The model under review builds one solid part; all positions refer to its coordinate system, in mm. A direction names the side the tool comes from. Coordinates: 2 decimals unless noted, no trailing zeros. Loops run counter-clockwise (first coordinate to the right, second up) from the corner with the lowest first, then second, coordinate; pieces in that order, holes last. Notation, with made-up numbers: M 88.25,-19.5 L 99.25,-19.5 A15 cw 99.25,8.5 Z; hole C 76.5,-8 d10. An arc over 180 degrees is marked long. Write item = value, one per line. Start each with the question number.
Q1. Clearance check with flat-ended pins moving along their axes: pin 1 Ø5 at (x, y) = (39, 3) entering from +Z; pin 2 Ø10 at (x, z) = (27, 9) entering from +Y; pin 3 Ø9.5 at (x, z) = (71, 0.5) entering from -Y. State where each tip first meets the part, or that it passes through.
Q2. For faces 4 (the face through (77, 19, 6.5)), 5 (the face through (-8, -5, 9)), 6 (the face through (-15.62, 14.6, -3.47)), 7 (the face through (36, 5, -6.5)), list the 3-axis set-ups (+Z, -Z, +X, -X, +Y, -Y) from which the entire face can be reached by the end or side of a thin tool; tool diameter is ignored.
Q3. Mouldability with a two-part tool opening along X and no side actions: class faces 1 (the face through (28.885, 8.019, 5.899)), 2 (the face through (78.64, 23.09, -0.09)), 3 (the face through (0, 0, -13)) as released by +X, released by -X, zero draft, split by the parting line, or undercut.
Q4. We need section A-A on y = -20.5. Give the boundary of the cut face in (x, z).
Q5. We need section C-C on y = 32.5. Give the boundary of the cut face in (x, z), and give its area (3 significant figures).
Q6. Wall thickness on probe 1 along X at (y, z) = (19, 0); probe 2 along X at (y, z) = (16, 0); probe 3 along Y at (x, z) = (0, 3): over which ranges is each line inside the solid? List them lowest first.
Q7. We need section B-B on y = 83. Give the boundary of the cut face in (x, z).
from build123d import *

# Parameters (mm, degrees)
SKETCH1_R           = 21
BOSS_EXTRUDE1_DEPTH = 22
SKETCH3_W           = 35
SKETCH3_H           = 18
BOSS_EXTRUDE2_DEPTH = 15
BOSS_EXTRUDE3_DEPTH = 9
SKETCH6_R           = 12.5
CUT_EXTRUDE1_DEPTH  = 18
BOSS_EXTRUDE5_DEPTH = 6.5
SKETCH9_R           = 20
BOSS_EXTRUDE6_DEPTH = 55
SKETCH10_R          = 22.5
BOSS_EXTRUDE7_DEPTH = 33
FILLET1_R           = 15
CHAMFER2_SIZE       = 10
FILLET3_R           = 2
FILLET4_R           = 2
FILLET5_R           = 2
CUT_EXTRUDE4_DEPTH  = 25
SKETCH13_R          = 16
CUT_EXTRUDE6_DEPTH  = 15


with BuildPart() as part:
    # Sketch1 → Boss-Extrude1 (new body)
    with BuildSketch(Plane(origin=(0, 0, 0), x_dir=(1, 0, 0), z_dir=(0, 1, 0))):
        with Locations(Location((0, 0, 0), (0, 0, 270))):
            Circle(SKETCH1_R)
    extrude(amount=BOSS_EXTRUDE1_DEPTH)

    # Sketch3 → Boss-Extrude2 (add)
    with BuildSketch(Plane.XZ):
        Rectangle(SKETCH3_W, SKETCH3_H)
    extrude(amount=BOSS_EXTRUDE2_DEPTH)

    # Sketch5 → Boss-Extrude3 (add, symmetric)
    with BuildSketch(Plane.XY):
        with BuildLine():
            Line((-17.5, -15), (17.5, -15))
            ThreePointArc((17.5, -15), (0, -32.5), (-17.5, -15))
        make_face()
    extrude(amount=BOSS_EXTRUDE3_DEPTH, both=True)

    # Sketch6 → Cut-Extrude1 (cut)
    with BuildSketch(Plane(origin=(0, 0, -9), x_dir=(-1, 0, 0), z_dir=(0, 0, -1))):
        with Locations((0, -15)):
            Circle(SKETCH6_R)
    extrude(amount=-CUT_EXTRUDE1_DEPTH, mode=Mode.SUBTRACT)

    # Sketch7 → Boss-Extrude5 (add, symmetric)
    with BuildSketch(Plane.XY):
        Polygon((17.5, -7.5), (88.273330058, 17.322081953), (84.484801337, 28.124028145), (17.5, 4.63068359), align=None)
    extrude(amount=BOSS_EXTRUDE5_DEPTH, both=True)

    # Sketch9 → Boss-Extrude6 (add)
    with BuildSketch(Plane(origin=(0, 12, 0), x_dir=(1, 0, 0), z_dir=(0, 1, 0))):
        with Locations(Location((55.484801337, 0, 0), (0, 0, 270))):
            Circle(SKETCH9_R)
    extrude(amount=BOSS_EXTRUDE6_DEPTH)

    # Sketch10 → Boss-Extrude7 (add)
    with BuildSketch(Plane(origin=(0, 67, 0), x_dir=(1, 0, 0), z_dir=(0, 1, 0))):
        with Locations(Location((55.484801337, 0, 0), (0, 0, 270))):
            Circle(SKETCH10_R)
    extrude(amount=BOSS_EXTRUDE7_DEPTH)

    # Fillet1
    # the kernel refuses this fillet: 15 mm, written as the material it takes off along each edge
    with BuildSketch(Plane(origin=(55.484801337, 67, 0), x_dir=(0, 0, 1), z_dir=(-1, 0, 0))) as fillet1_piece_1:
        with BuildLine():
            CenterArc((7.5, 8.291561976), FILLET1_R, 326.442690238, 33.557309762)
            Line((20, 0), (20.25, -0.16583124))
            ThreePointArc((20.25, -0.16583124), (21.25, -0.3), (22.5, -0.3))
            Line((22.5, -0.3), (22.8, 0))
            Line((22.8, 0), (22.8, 8.291561976))
            Line((22.8, 8.291561976), (22.5, 8.291561976))
        make_face()
    revolve(axis=Axis((55.484801337, 67, 0), (0, 1, 0)), mode=Mode.SUBTRACT)

    # Chamfer2
    # the kernel refuses this chamfer: 10 mm, written as the material it takes off along each edge
    with BuildSketch(Plane(origin=(84.484801337, 28.124028145, -32.21682988), x_dir=(-0.9523876901556013, -0.30488963189993584, 0), z_dir=(0, 0, 1))) as chamfer2_piece_1_section:
        Polygon((CHAMFER2_SIZE * 0.999621916911, CHAMFER2_SIZE * 0.0274958766106), (-CHAMFER2_SIZE * 0.0274958766106, CHAMFER2_SIZE * 0.999621916911), (0, 0), align=None)
    chamfer2_piece_1 = extrude(amount=64.433659759, mode=Mode.PRIVATE)
    chamfer2_piece_1 = chamfer2_piece_1 - Plane(origin=(55.484801337, 23.91959175, 0), x_dir=(0, 0, 1), z_dir=(0, -1, 0)) * Cylinder(20, 169, mode=Mode.PRIVATE)
    add(chamfer2_piece_1, mode=Mode.SUBTRACT)
    with BuildSketch(Plane(origin=(88.273330058, 17.322081953, -32.21682988), x_dir=(-0.9341875594200248, -0.3567822919160335, 0), z_dir=(0, 0, 1))) as chamfer2_piece_2:
        Polygon((CHAMFER2_SIZE * 0.999621916911, -CHAMFER2_SIZE * 0.0274958766106), (-CHAMFER2_SIZE * 0.0274958766106, -CHAMFER2_SIZE * 0.999621916911), (0, 0), align=None)
    extrude(amount=64.433659759, mode=Mode.SUBTRACT)

    # Fillet3
    fillet3_edges = [part.edges().sort_by_distance(p)[0] for p in [
        (45.299439603, 2.25, -6.5),
        (29.240150797, 8.748265524, -6.5),
        (29.240150797, 8.748265524, 6.5),
        (45.299439603, 2.25, 6.5),
    ]]
    fillet(fillet3_edges, radius=FILLET3_R)

    # Fillet4
    # the kernel refuses this fillet: 2 mm, written as the material it takes off along each edge
    with BuildSketch(Plane(origin=(0, 0, 0), x_dir=(0.9971250818764672, 0, -0.07577315548958338), z_dir=(0.07577315548958338, 0, 0.9971250818764672))) as fillet4_piece_1_section:
        with BuildLine():
            CenterArc((21 - FILLET4_R, FILLET4_R), FILLET4_R, 270, 90)
            Line((21 - FILLET4_R, 0), (21, 0))
            Line((21, 0), (21, FILLET4_R))
        make_face()
    fillet4_piece_1 = revolve(axis=Axis((0, 0, 0), (0, 1, 0)), revolution_arc=265.654352731, mode=Mode.PRIVATE)
    fillet4_piece_1 = split(fillet4_piece_1, bisect_by=Plane(origin=(19.021746519, 0.448100529, -6.5), z_dir=(0, 0, -1)), keep=Keep.TOP, mode=Mode.PRIVATE)
    fillet4_piece_1 = split(fillet4_piece_1, bisect_by=Plane(origin=(17.5, 0.448100529, -7.756660991), z_dir=(1, 0, 0)), keep=Keep.TOP, mode=Mode.PRIVATE)
    add(fillet4_piece_1, mode=Mode.SUBTRACT)
    with BuildSketch(Plane(origin=(0, 0, 0), x_dir=(0.9971250818764672, 0, -0.07577315548958338), z_dir=(0.07577315548958338, 0, 0.9971250818764672))) as fillet4_piece_2_section:
        with BuildLine():
            CenterArc((21 - FILLET4_R, FILLET4_R), FILLET4_R, 270, 90)
            Line((21 - FILLET4_R, 0), (21, 0))
            Line((21, 0), (21, FILLET4_R))
        make_face()
    fillet4_piece_2 = revolve(axis=Axis((0, 0, 0), (0, 1, 0)), revolution_arc=265.654352731, mode=Mode.PRIVATE)
    fillet4_piece_2 = split(fillet4_piece_2, bisect_by=Plane(origin=(0, 0.562448444, -9), z_dir=(0, 0, -1)), keep=Keep.TOP, mode=Mode.PRIVATE)
    add(fillet4_piece_2, mode=Mode.SUBTRACT)
    with BuildSketch(Plane(origin=(0, 0, 0), x_dir=(0.9971250818764672, 0, -0.07577315548958338), z_dir=(0.07577315548958338, 0, 0.9971250818764672))) as fillet4_piece_3_section:
        with BuildLine():
            CenterArc((21 - FILLET4_R, FILLET4_R), FILLET4_R, 270, 90)
            Line((21 - FILLET4_R, 0), (21, 0))
            Line((21, 0), (21, FILLET4_R))
        make_face()
    fillet4_piece_3 = revolve(axis=Axis((0, 0, 0), (0, 1, 0)), revolution_arc=265.654352731, mode=Mode.PRIVATE)
    fillet4_piece_3 = split(fillet4_piece_3, bisect_by=Plane(origin=(-17.5, 0.448099897, -7.756661101), z_dir=(-1, 0, 0)), keep=Keep.TOP, mode=Mode.PRIVATE)
    add(fillet4_piece_3, mode=Mode.SUBTRACT)
    with BuildSketch(Plane(origin=(0, 0, 0), x_dir=(0.9971250818764672, 0, -0.07577315548958338), z_dir=(0.07577315548958338, 0, 0.9971250818764672))) as fillet4_piece_4_section:
        with BuildLine():
            CenterArc((21 - FILLET4_R, FILLET4_R), FILLET4_R, 270, 90)
            Line((21 - FILLET4_R, 0), (21, 0))
            Line((21, 0), (21, FILLET4_R))
        make_face()
    fillet4_piece_4 = revolve(axis=Axis((0, 0, 0), (0, 1, 0)), revolution_arc=265.654352731, mode=Mode.PRIVATE)
    fillet4_piece_4 = split(fillet4_piece_4, bisect_by=Plane(origin=(-10.643200487, 0.567263166, 9), z_dir=(0, 0, 1)), keep=Keep.TOP, mode=Mode.PRIVATE)
    add(fillet4_piece_4, mode=Mode.SUBTRACT)
    with BuildSketch(Plane(origin=(0, 0, 0), x_dir=(0, 0, 1), z_dir=(-1, 0, 0))) as fillet4_piece_5_section:
        with BuildLine():
            CenterArc((21 - FILLET4_R, FILLET4_R), FILLET4_R, 270, 90)
            Line((21 - FILLET4_R, 0), (21, 0))
            Line((21, 0), (21, FILLET4_R))
        make_face()
    fillet4_piece_5 = revolve(axis=Axis((0, 0, 0), (0, 1, 0)), revolution_arc=85.61482077, mode=Mode.PRIVATE)
    fillet4_piece_5 = split(fillet4_piece_5, bisect_by=Plane(origin=(10.643200508, 0.567263125, 9), z_dir=(0, 0, 1)), keep=Keep.TOP, mode=Mode.PRIVATE)
    add(fillet4_piece_5, mode=Mode.SUBTRACT)
    with BuildSketch(Plane(origin=(0, 0, 0), x_dir=(0, 0, 1), z_dir=(-1, 0, 0))) as fillet4_piece_6_section:
        with BuildLine():
            CenterArc((21 - FILLET4_R, FILLET4_R), FILLET4_R, 270, 90)
            Line((21 - FILLET4_R, 0), (21, 0))
            Line((21, 0), (21, FILLET4_R))
        make_face()
    fillet4_piece_6 = revolve(axis=Axis((0, 0, 0), (0, 1, 0)), revolution_arc=85.61482077, mode=Mode.PRIVATE)
    fillet4_piece_6 = split(fillet4_piece_6, bisect_by=Plane(origin=(19.021746751, 0.448100278, 6.5), z_dir=(0, 0, 1)), keep=Keep.TOP, mode=Mode.PRIVATE)
    fillet4_piece_6 = split(fillet4_piece_6, bisect_by=Plane(origin=(17.5, 0.448100278, 7.756660688), z_dir=(1, 0, 0)), keep=Keep.TOP, mode=Mode.PRIVATE)
    add(fillet4_piece_6, mode=Mode.SUBTRACT)

    # Fillet5
    fillet5_edges = [part.edges().sort_by_distance(p)[0] for p in [
        (55.484801337, 100, -22.5),
    ]]
    fillet(fillet5_edges, radius=FILLET5_R)

    # Sketch12 → Cut-Extrude4 (cut, symmetric)
    with BuildSketch(Plane(origin=(55, 0, 0), x_dir=(0, 0, -1), z_dir=(1, 0, 0))):
        Polygon((6.5, 12), (20, 29.283691076), (20, 12), align=None)
        Polygon((-20, 12), (-6.5, 12), (-20, 29.283691076), align=None)
    extrude(amount=CUT_EXTRUDE4_DEPTH, both=True, mode=Mode.SUBTRACT)

    # Sketch13 → Cut-Extrude6 (cut)
    with BuildSketch(Plane(origin=(0, 22, 0), x_dir=(1, 0, 0), z_dir=(0, 1, 0))):
        with Locations(Location((0, 0, 0), (0, 0, 270))):
            Circle(SKETCH13_R)
    extrude(amount=-CUT_EXTRUDE6_DEPTH, mode=Mode.SUBTRACT)


solid = part.part
Returned:
q1.pin_1 = 6.5
q1.pin_2 = 8.97
q1.pin_3 = 9.6
q2.face_4 = +Z, +X, -Y
q2.face_5 = +Z, +X, -X, -Y
q2.face_6 = +Y
q2.face_7 = -Z, +X, -Y
q3.face_1 = undercut
q3.face_2 = released by +X
q3.face_3 = zero draft
q4.outline = M -16.61,-9 L -11.22,-9 L -11.22,9 L -16.61,9 Z; M 11.22,-9 L 16.61,-9 L 16.61,9 L 11.22,9 Z
q5.outline = C 55.48,0 d40
q5.area = 1,260 mm^2
q6.probe_1 = -21 to -16, 16 to 21, 35.48 to 81.23
q6.probe_2 = -21 to -16, 16 to 21, 35.48 to 79.79
q6.probe_3 = -32.5 to -27.5, -2.5 to 7
q7.outline = C 55.48,0 d45
